Geometry: final body of the model. Coordinates: model frame, mm. Face numbers are marked on the shaded views. Round coordinates to 2 decimals unless told otherwise and drop trailing zeros. Loops run counter-clockwise (first coordinate to the right, second up) from the corner with the lowest first, then second, coordinate; pieces in that order, holes last. Notation, with made-up numbers: (11, 83) -> (49, 83) arc R33 cw to (49, 114) -> close; hole circle Ø9 at (58.5, 3). An arc over 180 degrees is marked (long way). Answer in a Markdown table with one row per item.
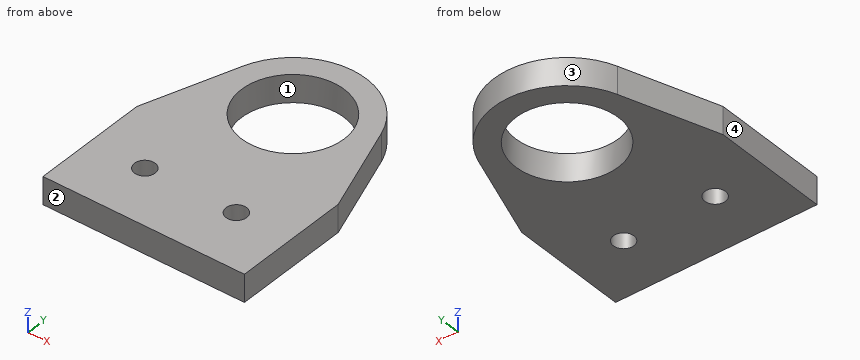
```python
from build123d import *

# Parameters (mm, degrees)
SKETCH1_R            = 11.2
SKETCH1_W            = 44
SKETCH1_H            = 25.4
BOSS_EXTRUDE1_DEPTH  = 6
M4_CLEARANCE_HOLE1_D = 4.5


with BuildPart() as part:
    # Sketch1 → Boss-Extrude1 (new body)
    # profile 1 of 2: a face of its own
    with BuildSketch(Plane.XY):
        with BuildLine():
            ThreePointArc((-15.148252746, 5.150770694), (0, 16), (15.148252746, 5.150770694))
            Line((15.148252746, 5.150770694), (22, -15))
            Line((22, -15), (-22, -15))
            Line((-22, -15), (-15.148252746, 5.150770694))
        make_face()
        Circle(SKETCH1_R, mode=Mode.SUBTRACT)
    # profile 2 of 2: a face of its own
    with BuildSketch(Plane.XY):
        with Locations((0, -27.7)):
            Rectangle(SKETCH1_W, SKETCH1_H)
    extrude(amount=BOSS_EXTRUDE1_DEPTH)

    # M4 Clearance Hole1 (through all)
    with Locations(Plane.XY.offset(6)):
        with Locations((-10, -27.7), (10, -27.7)):
            Hole(M4_CLEARANCE_HOLE1_D / 2)


solid = part.part
```
Item 1: Cut plane B-B (x = 0). Output: boundary loops of the cut face in (y, z).
Answer:
| item | result |
|---|---|
| outline | (-40.4, 0) -> (-11.2, 0) -> (-11.2, 6) -> (-40.4, 6) -> close; (11.2, 0) -> (16, 0) -> (16, 6) -> (11.2, 6) -> close |
Item 2: Draft query along X for the marked faces 1, 2, 3 and 4. Return one class per face: pulls with the +X half, pulls with the -X half, needs draft (parallel to the pull), parting line crosses it, or undercut.
Answer:
| item | result |
|---|---|
| face 1 | undercut |
| face 2 | needs draft |
| face 3 | parting line crosses it |
| face 4 | pulls with the -X half |
Item 3: Line query: probe 1 along Y at (x, z) = (-10, 3.75); probe 2 along Y at (x, z) = (0, 3.65); probe 3 along X at (y, z) = (-3.5, 1.1). Output: solid intervals per line, ascending. Write a range as [from, to].
Answer:
| item | result |
|---|---|
| probe 1 | y = [-40.4, -29.95], [-25.45, -5.04], [5.04, 12.49] |
| probe 2 | y = [-40.4, -11.2], [11.2, 16] |
| probe 3 | x = [-18.09, -10.64], [10.64, 18.09] |
Item 4: Cut plane D-D (x = 10). Output: boundary loops of the cut face in (y, z).
Answer:
| item | result |
|---|---|
| outline | (-40.4, 0) -> (-29.95, 0) -> (-29.95, 6) -> (-40.4, 6) -> close; (-25.45, 0) -> (-5.04, 0) -> (-5.04, 6) -> (-25.45, 6) -> close; (5.04, 0) -> (12.49, 0) -> (12.49, 6) -> (5.04, 6) -> close |
Item 5: Pin query (flat end, axial travel): pin 1 Ø1 at (x, z) = (-13, 2.5) entering from +Y; pin 2 Ø3 at (y, z) = (-8, 0.5) entering from -X. Return the tip coordinate at first contact, or that it passes through.
Answer:
| item | result |
|---|---|
| pin 1 | stops at y = 9.99 |
| pin 2 | stops at x = -20.13 |
Item 6: Cut plane C-C (z = 3.8). Output: boundary loops of the cut face in (x, y).
Answer:
| item | result |
|---|---|
| outline | (-22, -40.4) -> (22, -40.4) -> (22, -15) -> (15.15, 5.15) arc R16 ccw to (-15.15, 5.15) -> (-22, -15) -> close; hole circle Ø4.5 at (-10, -27.7); hole circle Ø22.4 at (0, 0); hole circle Ø4.5 at (10, -27.7) |
Item 7: Cut plane A-A (y = -27.7). Output: boundary loops of the cut face in (x, z), then the cut area to 3 significant figures.
Answer:
| item | result |
|---|---|
| outline | (-22, 0) -> (-12.25, 0) -> (-12.25, 6) -> (-22, 6) -> close; (-7.75, 0) -> (7.75, 0) -> (7.75, 6) -> (-7.75, 6) -> close; (12.25, 0) -> (22, 0) -> (22, 6) -> (12.25, 6) -> close |
| area | 210 mm² |
